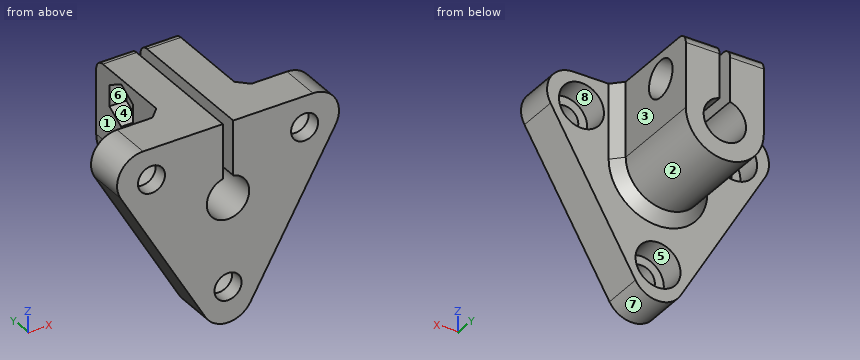
```python
from build123d import *

# Parameters (mm, degrees)
ESQUISSE5_R              = 2.6
BOSS_EXTRU_2_DEPTH       = 7.8
ESQUISSE6_R              = 7.5
BOSS_EXTRU_3_DEPTH       = 20
BOSS_EXTRU_6_START       = -20
BOSS_EXTRU_6_DEPTH       = 20
ESQUISSE14_R             = 4.075
ENL_V_MAT_EXTRU_4_DEPTH  = 48.235297536
ENL_V_MAT_EXTRU_5_DEPTH  = 48.235297536
CONG_2_R                 = 5
ESQUISSE17_R             = 2.075
ENL_V_MAT_EXTRU_6_DEPTH  = 47.62863011
ENL_V_MAT_EXTRU_7_DEPTH  = 3.25
ESQUISSE19_R             = 4.325
ENL_V_MAT_EXTRU_8_DEPTH  = 5
ESQUISSE20_R             = 3.525
ENL_V_MAT_EXTRU_9_DEPTH  = 4.97
CONG_3_R                 = 2
CHANFREIN2_SIZE          = 2
ENL_V_MAT_EXTRU_10_DEPTH = 44.729429119


with BuildPart() as part:
    # Esquisse5 → Boss.-Extru.2 (new body)
    with BuildSketch(Plane(origin=(0, 0, 0), x_dir=(1, 0, 0), z_dir=(0, 1, 0))):
        Polygon((-25, -14.43375673), (25, -14.43375673), (0, 28.867513459), align=None)
        with Locations(Location((0, 17, 0), (0, 0, 270))):
            Circle(ESQUISSE5_R, mode=Mode.SUBTRACT)
        with Locations(Location((-14.722431864, -8.5, 0), (0, 0, 270))):
            Circle(ESQUISSE5_R, mode=Mode.SUBTRACT)
        with Locations(Location((14.722431864, -8.5, 0), (0, 0, 270))):
            Circle(ESQUISSE5_R, mode=Mode.SUBTRACT)
    extrude(amount=BOSS_EXTRU_2_DEPTH)

    # Esquisse6 → Boss.-Extru.3 (add)
    with BuildSketch(Plane(origin=(0, 7.8, 0), x_dir=(1, 0, 0), z_dir=(0, 1, 0))):
        with Locations(Location((0, 0, 0), (0, 0, 270))):
            Circle(ESQUISSE6_R)
    extrude(amount=BOSS_EXTRU_3_DEPTH)

    # Esquisse13 → Boss.-Extru.6 (add)
    with BuildSketch(Plane(origin=(0, 27.8, 0), x_dir=(1, 0, 0), z_dir=(0, 1, 0)).offset(BOSS_EXTRU_6_START)):
        with BuildLine():
            Line((-7.5, 0), (-7.5, -14.43375673))
            Line((-7.5, -14.43375673), (7.5, -14.43375673))
            Line((7.5, -14.43375673), (7.5, 0))
            ThreePointArc((7.5, 0), (0, -7.5), (-7.5, 0))
        make_face()
    extrude(amount=BOSS_EXTRU_6_DEPTH)

    # Esquisse14 → Enlèv. mat.-Extru.4 (cut, through all)
    with BuildSketch(Plane(origin=(0, 27.8, 0), x_dir=(1, 0, 0), z_dir=(0, 1, 0))):
        with Locations(Location((0, 0, 0), (0, 0, 270))):
            Circle(ESQUISSE14_R)
    extrude(amount=-ENL_V_MAT_EXTRU_4_DEPTH, mode=Mode.SUBTRACT)

    # Esquisse15 → Enlèv. mat.-Extru.5 (cut, through all)
    with BuildSketch(Plane(origin=(0, 27.8, 0), x_dir=(1, 0, 0), z_dir=(0, 1, 0))):
        with BuildLine():
            Line((-1, -3.95039555), (-1, -14.43375673))
            Line((-1, -14.43375673), (1, -14.43375673))
            Line((1, -14.43375673), (1, -3.95039555))
            ThreePointArc((1, -3.95039555), (0, -4.075), (-1, -3.95039555))
        make_face()
    extrude(amount=-ENL_V_MAT_EXTRU_5_DEPTH, mode=Mode.SUBTRACT)

    # Congé2
    cong_2_edges = [part.edges().sort_by_distance(p)[0] for p in [
        (0, 3.9, -28.867513459),
        (25, 3.9, 14.43375673),
        (-25, 3.9, 14.43375673),
    ]]
    fillet(cong_2_edges, radius=CONG_2_R)

    # Esquisse17 → Enlèv. mat.-Extru.6 (cut, through all)
    with BuildSketch(Plane(origin=(7.5, 0, 0), x_dir=(0, 0, -1), z_dir=(1, 0, 0))):
        with Locations((-9.43375673, 20.3)):
            Circle(ESQUISSE17_R)
    extrude(amount=-ENL_V_MAT_EXTRU_6_DEPTH, mode=Mode.SUBTRACT)

    # Esquisse18 → Enlèv. mat.-Extru.7 (cut)
    with BuildSketch(Plane.ZY.offset(7.5)):
        Polygon((11.468916429, 23.825), (7.398597031, 23.825), (5.363437332, 20.3), (7.398597031, 16.775), (11.468916429, 16.775), (13.504076128, 20.3), align=None)
    extrude(amount=-ENL_V_MAT_EXTRU_7_DEPTH, mode=Mode.SUBTRACT)

    # Esquisse19 → Enlèv. mat.-Extru.8 (cut)
    with BuildSketch(Plane(origin=(0, 7.8, 0), x_dir=(1, 0, 0), z_dir=(0, 1, 0))):
        with Locations(Location((0, 17, 0), (0, 0, 270))):
            Circle(ESQUISSE19_R)
        with Locations(Location((14.722431864, -8.5, 0), (0, 0, 270))):
            Circle(ESQUISSE19_R)
        with Locations(Location((-14.722431864, -8.5, 0), (0, 0, 270))):
            Circle(ESQUISSE19_R)
    extrude(amount=-ENL_V_MAT_EXTRU_8_DEPTH, mode=Mode.SUBTRACT)

    # Esquisse20 → Enlèv. mat.-Extru.9 (cut)
    with BuildSketch(Plane(origin=(7.5, 0, 0), x_dir=(0, 0, -1), z_dir=(1, 0, 0))):
        with Locations((-9.43375673, 20.3)):
            Circle(ESQUISSE20_R)
    extrude(amount=-ENL_V_MAT_EXTRU_9_DEPTH, mode=Mode.SUBTRACT)

    # Congé3
    cong_3_edges = [part.edges().sort_by_distance(p)[0] for p in [
        (-4.25, 27.8, 14.43375673),
        (4.25, 27.8, 14.43375673),
    ]]
    fillet(cong_3_edges, radius=CONG_3_R)

    # Chanfrein2
    chanfrein2_edges = [part.edges().sort_by_distance(p)[0] for p in [
        (0, 7.8, -7.5),
        (7.5, 7.8, 7.216878365),
        (-7.5, 7.8, 7.216878365),
    ]]
    chamfer(chanfrein2_edges, length=CHANFREIN2_SIZE)

    # Esquisse21 → Enlèv. mat.-Extru.10 (cut, through all)
    with BuildSketch(Plane(origin=(2.53, 0, 0), x_dir=(0, 0, -1), z_dir=(1, 0, 0))):
        Polygon((-10.392924593, 22.140005981), (-8.474588866, 22.140005981), (-9.43375673, 22.640005981), align=None)
    extrude(amount=-ENL_V_MAT_EXTRU_10_DEPTH, mode=Mode.SUBTRACT)


solid = part.part
```
Source: CAD feature listing. Evaluate the final solid. Frame: model axes, mm. Face numbers are marked on the shaded views. A direction names the side the tool comes from. Give positions to 0.01 mm unless a question says otherwise; leave off trailing zeros. Write each loop counter-clockwise with the first axis right and the second up, starting at its lowest first coordinate (ties: lowest second). Pieces come first, ordered by that corner, then holes. Notation, with made-up numbers: (83.5, 40.5) - (132.5, 40.5) arc R5 ccw to (132.5, 47.5) - close; hole circle Ø3 at (-26, -11). An arc over 180 degrees is marked (long way). One line per item, written item: value. Start each with the question number.
Q1. Section query C-C, the plane z = -17. Return the cut outline in (x, y) (3 decimals), then the cut area to 3 significant figures.
Q2. Material intervals for probe 1 along X at (y, z) = (21.75, 0) (3 decimals); probe 2 along X at (y, z) = (18, 9.5); probe 3 along Z at (x, y) = (-2, 6.25), sorted ascending. Write a range as from..to.
Q3. Section query B-B, the plane y = 13.5. Return the cut outline in (x, z) (3 decimals).
Q4. Draft query along X for the marked faces 6, 7 and 8. Return one class per face: +X half, -X half, draft (parallel to the pull), parting line (faces both ways), or undercut.
Q5. First-contact query: pin 1 Ø3.5 at (y, z) = (20.5, 8) entering from +X; pin 2 Ø1.5 at (x, z) = (-11.5, -4.5) entering from +Y; pin 3 Ø1.5 at (y, z) = (17.5, -5.5) entering from -X. Flat tips, straight axial feed; report the tip coordinate or a pass-through.
Q6. Set-up query: the marked faces 1, 2, 3, 4 and 5. Return all of +Z, -Z, +X, -X, +Y, -Y with unobstructed straight access to the full face (end or side cutting, diameter ignored); none if empty.
Q7. Section query D-D, the plane y = 19.5. Return the cut outline in (x, z) (3 decimals), then the cut area to 3 significant figures.
Q8. Section query A-A, the plane x = 0. Return the cut outline in (y, z) (3 decimals), then the cut area to 3 significant figures.
Answer:
1. outline: (-6.852, 0) - (-2.6, 0) - (-2.6, 2.8) - (-4.325, 2.8) - (-4.325, 7.8) - (-6.852, 7.8) - close; (2.6, 0) - (6.852, 0) - (6.852, 7.8) - (4.325, 7.8) - (4.325, 2.8) - (2.6, 2.8) - close
1. area: 49.1 mm2
2. probe 1: x = -7.5..-4.075, 4.075..7.5
2. probe 2: x = -4.25..-1, 1..2.53
2. probe 3: z = -23.45..-20.83, -13.17..-3.55, 3.55..14.43
3. outline: (-7.5, 0) arc R7.5 ccw to (7.5, 0) - (7.5, 14.434) - (1, 14.434) - (1, 3.95) arc R4.075 cw (long way) to (-1, 3.95) - (-1, 14.434) - (-7.5, 14.434) - close
4. face 6: draft
4. face 7: parting line
4. face 8: undercut
5. pin 1: stops at x = 2.53
5. pin 2: stops at y = 7.8
5. pin 3: stops at x = -5.8
6. face 1: +Z, -Z, -X, +Y
6. face 2: -Z, +Y
6. face 3: +Z, -Z, +X, +Y
6. face 4: -X
6. face 5: +Y
7. outline: (-7.5, 0) arc R7.5 ccw to (7.5, 0) - (7.5, 6.001) - (2.53, 6.001) - (2.53, 7.519) - (1, 7.519) - (1, 3.95) arc R4.075 cw (long way) to (-1, 3.95) - (-1, 7.519) - (-4.25, 7.519) - (-4.25, 5.825) - (-7.5, 5.825) - close; (-7.5, 13.042) - (-4.25, 13.042) - (-4.25, 11.348) - (-1, 11.348) - (-1, 14.434) - (-7.5, 14.434) - close; (1, 11.348) - (2.53, 11.348) - (2.53, 12.867) - (7.5, 12.867) - (7.5, 14.434) - (1, 14.434) - close
7. area: 156 mm2
8. outline: (0, -23.868) - (7.8, -23.868) - (7.8, -21.325) - (2.8, -21.325) - (2.8, -19.6) - (0, -19.6) - close; (0, -14.4) - (2.8, -14.4) - (2.8, -12.675) - (7.8, -12.675) - (7.8, -9.5) - (9.8, -7.5) - (27.8, -7.5) - (27.8, -4.075) - (0, -4.075) - close
8. area: 167 mm2
